The model under review builds one solid part; all positions refer to its coordinate system, in mm. Face numbers are marked on the shaded views. A direction names the side the tool comes from. Round coordinates to 2 decimals unless told otherwise and drop trailing zeros. Order: outer loops, then holes, each group sorted by start corner. A loop starts at its lowest first (then second) coordinate and runs counter-clockwise, first axis right, second up. Notation, with made-up numbers: (-31.75, -2) -> (-16.75, -2) arc R29 cw to (-16.75, 36) -> close; hole circle Ø8 at (22, 12). An arc over 180 degrees is marked (long way). Use a Markdown table: item, result. Add a question column.
Autodesk Fusion 360 part; units mm, degrees
sketch "Sketch1" plane through (0, 0, 0) normal (0, 0, 1) x (1, 0, 0)
  circle A0 centre (0, 0) radius 10
  line L0 (0, 0) -> (0, 10) construction
  line L1 (0, 10) -> (0, 25)
  line L2 (0, 25) -> (-20, 25)
  line L3 (-20, 25) -> (-20, -25)
  line L4 (-20, -25) -> (0, -25)
  line L5 (0, -25) -> (0, -10)
  line L6 (-20, -25) -> (-20, -110)
  line L7 (-20, -110) -> (-10, -110)
  line L8 (-10, -110) -> (-10, -25)
  line L9 (-10, -25) -> (9, -25)
  line L10 (9, -25) -> (9, -40)
  line L11 (9, -40) -> (-10, -40)
  line L12 (-10, -40) -> (-10, -25)
  dimension "d1" = 20
  dimension "d2" = 15
  dimension "d3" = 20
  dimension "d4" = 50
  dimension "d5" = 85
  dimension "d6" = 10
  dimension "d7" = 19
extrude "Extrude1" add sketch "Sketch1" along normal blind 60 contours A0 L1 L2 L3 L4 L5 L9
extrude "Extrude2" add sketch "Sketch1" along normal blind 30 contours L4 L8 L9 L10 L11 L12
extrude "Extrude3" add sketch "Sketch1" along normal blind 60 contours L4 L6 L7 L8 L12
sketch "Sketch2" plane through (-20, 0, 0) normal (-1, 0, 0) x (0, -1, 0)
  line L0 (-25, 0) -> (110, 0)
  line L1 (110, 0) -> (110, 60)
  line L2 (110, 60) -> (-25, 60)
  line L3 (-25, 60) -> (-25, 0)
  line L4 (-25, 60) -> (-17.5, 60) construction
  line L5 (-17.5, 60) -> (27.5, 60) construction
  line L6 (-17.5, 60) -> (-17.5, 45) construction
  circle A0 centre (-17.5, 15) radius 2.5
  line L7 (110, 30) -> (102.5, 30) construction
  line L8 (102.5, 30) -> (102.5, 46.25) construction
  circle A1 centre (102.5, 46.25) radius 2.5
  circle A2 centre (102.5, 53.75) radius 2.5
  line L9 (102.5, 53.75) -> (100, 53.75) construction
  line L10 (102.5, 46.25) -> (100, 46.25) construction
  line L11 (100, 53.75) -> (100, 46.25)
  line L12 (105, 53.75) -> (105, 46.25)
  circle A3 centre (102.5, 6.25) radius 2.5
  line L13 (105, 6.25) -> (105, 13.75)
  circle A4 centre (102.5, 13.75) radius 2.5
  line L14 (100, 6.25) -> (100, 13.75)
  circle A5 centre (17.5, 15) radius 2.5
  circle A6 centre (-17.5, 45) radius 2.5
  circle A7 centre (17.5, 45) radius 2.5
  line L15 (-17.5, 45) -> (17.5, 45) construction
  line L16 (-17.5, 15) -> (17.5, 15) construction
  line L17 (0, 15) -> (0, 45) construction
  circle A8 centre (0, 30) radius 2.5
  dimension "d14" = 7.5
  dimension "d15" = 45
  dimension "d16" = 15
  dimension "d23" = 7.5
  dimension "d24" = 16.25
  dimension "d25" = 5
  dimension "d28" = 0
  dimension "d29" = 7.5
  dimension "d34" = 35
  dimension "d35" = 30
  dimension "d36" = 5
extrude "Extrude4" cut sketch "Sketch2" against normal blind 20 contours A0 | A1 | A1 A2 L11 L12 | A2 | A3 | A3 L13 A4 L14 | A4 | A5 | A6 | A7 | A8
sketch "Sketch3" plane through (-20, 0, 0) normal (-1, 0, 0) x (0, -1, 0)
  circle A0 centre (17.5, 45) radius 2.5
  circle A1 centre (-17.5, 45) radius 2.5
  circle A2 centre (17.5, 15) radius 2.5
  arc A3 (105, 13.75) -> (100, 13.75) centre (102.5, 13.75) ccw
  line L0 (105, 13.75) -> (105, 6.25)
  arc A4 (100, 6.25) -> (105, 6.25) centre (102.5, 6.25) ccw
  line L1 (100, 6.25) -> (100, 13.75)
  circle A5 centre (-17.5, 15) radius 2.5
  circle A6 centre (0, 30) radius 2.5
  arc A7 (100, 46.25) -> (105, 46.25) centre (102.5, 46.25) ccw
  line L2 (100, 46.25) -> (100, 53.75)
  arc A8 (105, 53.75) -> (100, 53.75) centre (102.5, 53.75) ccw
  line L3 (105, 53.75) -> (105, 46.25)
  line L4 (-25, 0) -> (110, 0)
  line L5 (110, 0) -> (110, 60)
  line L6 (110, 60) -> (-25, 60)
  line L7 (-25, 60) -> (-25, 0)
  circle A9 centre (-17.5, 45) radius 5
  circle A10 centre (17.5, 45) radius 5
  circle A11 centre (-17.5, 15) radius 5
  circle A12 centre (17.5, 15) radius 5
  line L8 (0, 30) -> (0, 35) construction
  line L9 (0, 35) -> (-4.3301, 32.5)
  line L10 (-4.3301, 32.5) -> (-4.3301, 27.5)
  line L11 (-4.3301, 27.5) -> (0, 25)
  line L12 (0, 25) -> (4.3301, 27.5)
  line L13 (4.3301, 27.5) -> (4.3301, 32.5)
  line L14 (4.3301, 32.5) -> (0, 35)
  point P0 (0, 30)
  dimension "d37" = 10
  dimension "d40" = 35
  dimension "d41" = -30
  dimension "d42" = 5
extrude "Extrude5" cut sketch "Sketch3" against normal blind 5 contours A9 | A10 | A11 | A12
extrude "Extrude6" cut sketch "Sketch3" against normal blind 6 from surface at -7 contours L9 L10 L11 L12 L13 L14
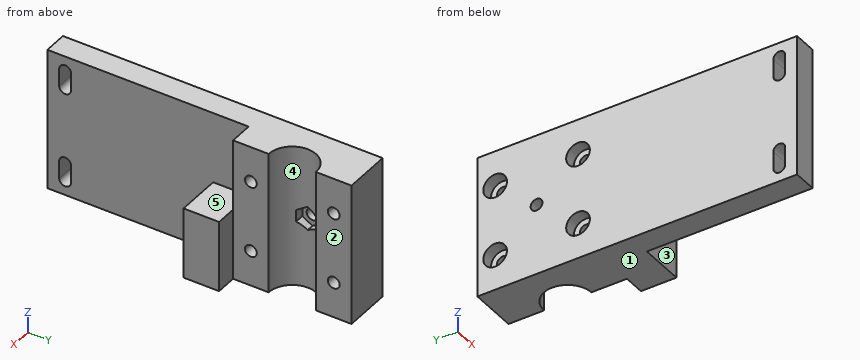
Q1. Add section D-D, the plane y = -17.5. Give the boundary of the cut face in (x, z).
Q2. To check wall thickness, follow line 1 along Z through (x, y) = (-10.75, 17.5); line 2 along Y through (x, z) = (-0.75, 10); line 3 along Y through (x, z) = (-11, 49). State the ranges of each line that lie inside material, in increasing order.
Q3. Add section A-A, the plane y = -102.5. Give the boundary of the cut face in (x, z), then the cut area to 3 significant figures.
Q4. Add section C-C, the plane z = 15. Give the number of separate pieces and of enclosed holes in the cut face, then the cut area to 3 significant figures.
Q5. Add section B-B, the plane x = -11.75. Give the boundary of the cut face in (y, z).
Q6. Draft analysis for pull direction Y (two halves, no side actions). For the marked faces 3, 4 and 5, state which applies: released by +Y, released by -Y, zero draft, split by the parting line, or undercut.
Q7. For the marked faces 1 and 2, list the 3-axis set-ups (+Z, -Z, +X, -X, +Y, -Y) from which the entire face can be reached by the end or side of a thin tool; tool diameter is ignored.
Q8. For pin 1 (5 mm diameter, centred on y = -18, z = 16, fed in from -X); pin 2 (8 mm diameter, centred on y = -16.5, z = 46, fed in from -X); pin 3 (3 mm diameter, centred on x = 1, z = 44.5, fed in from -Y); pin 4 (12 mm diameter, centred on x = -1, y = -48.5, fed in from -Z), all flat-tipped, find the tip position at first contact; note any pin that passes through.
Return value:
| question | item | result |
|---|---|---|
| 1 | outline | (-20, 0) -> (0, 0) -> (0, 12.5) -> (-15, 12.5) -> (-15, 10) -> (-20, 10) -> close; (-20, 20) -> (-15, 20) -> (-15, 17.5) -> (0, 17.5) -> (0, 42.5) -> (-15, 42.5) -> (-15, 40) -> (-20, 40) -> close; (-20, 50) -> (-15, 50) -> (-15, 47.5) -> (0, 47.5) -> (0, 60) -> (-20, 60) -> close |
| 2 | line 1 | 0 to 12.5, 17.5 to 42.5, 47.5 to 60 |
| 2 | line 2 | -40 to -9.97, 9.97 to 25 |
| 2 | line 3 | -110 to -105, -100 to 25 |
| 3 | outline | (-20, 0) -> (-10, 0) -> (-10, 3.75) -> (-20, 3.75) -> close; (-20, 16.25) -> (-10, 16.25) -> (-10, 43.75) -> (-20, 43.75) -> close; (-20, 56.25) -> (-10, 56.25) -> (-10, 60) -> (-20, 60) -> close |
| 3 | area | 350 mm² |
| 4 | separate pieces | 4 |
| 4 | enclosed holes | 0 |
| 4 | area | 1,680 mm² |
| 5 | outline | (-110, 0) -> (25, 0) -> (25, 60) -> (-110, 60) -> close; hole (-105, 6.25) arc R2.5 ccw to (-100, 6.25) -> (-100, 13.75) arc R2.5 ccw to (-105, 13.75) -> close; hole (-105, 46.25) arc R2.5 ccw to (-100, 46.25) -> (-100, 53.75) arc R2.5 ccw to (-105, 53.75) -> close; hole circle Ø5 at (-17.5, 15); hole circle Ø5 at (-17.5, 45); hole (-4.33, 27.5) -> (0, 25) -> (4.33, 27.5) -> (4.33, 32.5) -> (0, 35) -> (-4.33, 32.5) -> close; hole circle Ø5 at (17.5, 15); hole circle Ø5 at (17.5, 45) |
| 6 | face 3 | released by -Y |
| 6 | face 4 | undercut |
| 6 | face 5 | zero draft |
| 7 | face 1 | -Z, +X, -X, +Y, -Y |
| 7 | face 2 | +Z, -Z, +X, +Y |
| 8 | pin 1 | x = -15 |
| 8 | pin 2 | x = -20 |
| 8 | pin 3 | y = -25 |
| 8 | pin 4 | through |
